from build123d import *

# Parameters (mm, degrees)
SKETCH1_W               = 42
SKETCH1_H               = 30
BOSS_EXTRUDE1_DEPTH     = 4.5
BOSS_EXTRUDE2_DEPTH     = 10
FILLET1_R               = 6
SKETCH3_R               = 11.25
CUT_EXTRUDE1_DEPTH      = 3
CUT_EXTRUDE2_DEPTH      = 29.253318389
CUT_EXTRUDE2_DEPTH_BACK = 29.253318389
SKETCH4_R               = 7
FILLET2_R               = 2
CHAMFER1_SIZE           = 1
SKETCH6_R               = 2.15
CUT_EXTRUDE4_DEPTH      = 40.385911187
SKETCH7_R               = 1.5
CUT_EXTRUDE5_DEPTH      = 10


with BuildPart() as part:
    # Sketch1 → Boss-Extrude1 (new body)
    with BuildSketch(Plane.XY):
        Rectangle(SKETCH1_W, SKETCH1_H)
    extrude(amount=BOSS_EXTRUDE1_DEPTH)

    # Sketch2 → Boss-Extrude2 (add)
    with BuildSketch(Plane.XY.offset(4.5)):
        Polygon((21, -9), (10, -9), (10, -1.5), (7, -1.5), (7, -12), (-10.5, -12), (-10.5, -15), (21, -15), align=None)
    extrude(amount=BOSS_EXTRUDE2_DEPTH)

    # Fillet1
    fillet1_edges = [part.edges().sort_by_distance(p)[0] for p in [
        (10, -5.25, 4.5),
        (7, -12, 9.5),
    ]]
    fillet(fillet1_edges, radius=FILLET1_R)

    # Sketch3 → Cut-Extrude1 (cut)
    with BuildSketch(Plane(origin=(0, 0, 0), x_dir=(-1, 0, 0), z_dir=(0, 0, -1))):
        with Locations((0, -6.25)):
            Circle(SKETCH3_R)
    extrude(amount=-CUT_EXTRUDE1_DEPTH, mode=Mode.SUBTRACT)

    # Sketch4 → Cut-Extrude2 (cut, two sides: drawn at the far end of the back side and taken through both)
    with BuildSketch(Plane(origin=(0, 0, 3), x_dir=(-1, 0, 0), z_dir=(0, 0, -1)).offset(-CUT_EXTRUDE2_DEPTH_BACK)):
        with Locations((0, -6.25)):
            Circle(SKETCH4_R)
    extrude(amount=CUT_EXTRUDE2_DEPTH + CUT_EXTRUDE2_DEPTH_BACK, mode=Mode.SUBTRACT)

    # Fillet2
    fillet2_edges = [part.edges().sort_by_distance(p)[0] for p in [
        (21, -15, 7.25),
        (-21, -15, 2.25),
        (-21, 15, 2.25),
        (21, 15, 2.25),
    ]]
    fillet(fillet2_edges, radius=FILLET2_R)

    # Chamfer1
    chamfer1_edges = [part.edges().sort_by_distance(p)[0] for p in [
        (-10.5, -12, 9.5),
    ]]
    chamfer(chamfer1_edges, length=CHAMFER1_SIZE)

    # Sketch6 → Cut-Extrude4 (cut, through all)
    with BuildSketch(Plane.XZ.offset(15)):
        with Locations(Location((-6.35, 10.55, 0), (0, 0, 270))):
            Circle(SKETCH6_R)
    extrude(amount=-CUT_EXTRUDE4_DEPTH, mode=Mode.SUBTRACT)

    # Sketch7 → Cut-Extrude5 (cut)
    with BuildSketch(Plane.XY.offset(4.5)):
        with Locations((-15.5, 9.25)):
            Circle(SKETCH7_R)
        with Locations((15.5, 9.25)):
            Circle(SKETCH7_R)
    extrude(amount=-CUT_EXTRUDE5_DEPTH, mode=Mode.SUBTRACT)


solid = part.part
Verification items for the finished model (mm, model axes). A direction names the side the tool comes from. Give positions to 0.01 mm unless a question says otherwise; leave off trailing zeros. Loops run counter-clockwise (first coordinate to the right, second up) from the corner with the lowest first, then second, coordinate; pieces in that order, holes last.
1) Sectioned sample at A-A, the plane x = -15.5. Enter the section's corners in (y, z), then the cut area to 4 significant figures.
2) Sectioned sample at C-C, the plane x = -6.35. Enter the section's corners in (y, z), then the cut area to 3 significant figures.
3) Sectioned sample at B-B, the plane y = -10. Enter the section's corners in (x, z), then the cut area to 3 significant figures.
4) Set-up check for faces 4 (the flat face through (-10.5, -14, 9)), 5 (the flat face through (-5, 0, 3)), 6 (the flat face through (-10, -12.5, 9.4)): record each of +Z, -Z, +X, -X, +Y, -Y from which the full face is reachable in a straight line by a thin tool's end or side.
5) Depth check by flat-ended pin: pin 1 Ø5.5 at (x, z) = (-6.35, 10.55) entering from +Y; pin 2 Ø5 at (y, z) = (-3.5, 7.5) entering from -X; pin 3 Ø4.5 at (x, z) = (10, 8) entering from +Y; pin 4 Ø6 at (y, z) = (4, 8) entering from -X. Enter the tip coordinate at first touch or a pass-through.
6) Thickness scan on line 1 along Z through (x, y) = (9, -7.5); line 2 along Z through (x, y) = (8.5, 1.5); line 3 along X through (y, z) = (-13.6, 10.55). Record the ranges inside material, lowest first.
7) Draft check along X on faces 1 (the flat face through (9, -11, 14.5)), 2 (the cylindrical face through (1.517, -13.084, 7.553)), 3 (the cylindrical face through (11.804, -5.198, 6.211)). Enter one of: pulls with the +X half, pulls with the -X half, needs draft (parallel to the pull), parting line crosses it, or undercut.
8) Sectioned sample at D-D, the plane z = 5.75. Enter the section's corners in (x, y).
Answers:
1. outline: (-15, 0) - (7.75, 0) - (7.75, 4.5) - (-15, 4.5) - close; (10.75, 0) - (15, 0) - (15, 4.5) - (10.75, 4.5) - close
1. area: 121.5 mm2
2. outline: (-15, 3) - (-9.2, 3) - (-9.2, 4.5) - (-12, 4.5) - (-12, 8.4) - (-15, 8.4) - close; (-15, 12.7) - (-12, 12.7) - (-12, 14.5) - (-15, 14.5) - close; (-3.3, 3) - (3.04, 3) - (3.04, 0) - (15, 0) - (15, 4.5) - (-3.3, 4.5) - close
2. area: 89.2 mm2
3. outline: (-21, 0) - (-10.61, 0) - (-10.61, 3) - (-5.91, 3) - (-5.91, 4.5) - (-21, 4.5) - close; (5.91, 3) - (10.61, 3) - (10.61, 0) - (21, 0) - (21, 14.5) - (5.91, 14.5) - close
3. area: 259 mm2
4. face 4: +Z, -X, +Y, -Y
4. face 5: -Z
4. face 6: +Z, -X, +Y
5. pin 1: stops at y = -12
5. pin 2: stops at x = 7
5. pin 3: stops at y = -1.5
5. pin 4: passes through
6. line 1: z = 3 to 14.5
6. line 2: z = 0 to 4.5
6. line 3: x = -10.5 to -8.5, -4.2 to 20.91
7. face 1: needs draft
7. face 2: undercut
7. face 3: pulls with the +X half
8. outline: (-10.5, -15) - (19, -15) arc R2 ccw to (21, -13) - (21, -9) - (12.33, -9) - (12.33, -1.5) - (7, -1.5) - (7, -6) arc R6 cw to (7, -6.12) arc R7 cw to (-3.99, -12) - (-9.5, -12) - (-10.5, -13) - close
